from build123d import *

# Parameters (mm, degrees)
SKETCH1_R                 = 82
SKETCH1_R_2               = 75
BOSS_EXTRUDE1_DEPTH       = 9
SKETCH2_R                 = 5
CUT_EXTRUDE1_DEPTH        = 117.314229568
CIRPATTERN1_COUNT         = 4
M2X0_4_TAPPED_HOLE1_D     = 1.6
M2X0_4_TAPPED_HOLE1_DEPTH = 10
M2X0_4_TAPPED_HOLE1_TIP   = 0.480688495


with BuildPart() as part:
    # Sketch1 → Boss-Extrude1 (new body)
    with BuildSketch(Plane.XY):
        Circle(SKETCH1_R)
        Circle(SKETCH1_R_2, mode=Mode.SUBTRACT)
    extrude(amount=BOSS_EXTRUDE1_DEPTH)

    # Sketch2 → Cut-Extrude1 (cut, through all)
    with BuildSketch(Plane.XY.offset(9)):
        with Locations((0, 83)):
            Circle(SKETCH2_R)
    cut_extrude1 = extrude(amount=-CUT_EXTRUDE1_DEPTH, mode=Mode.SUBTRACT)

    # CirPattern1: Cut-Extrude1 ×4 about axis
    cirpattern1_axis = Axis((0, 0, 0), (0, 0, 1))
    for i in range(1, CIRPATTERN1_COUNT):
        add(cut_extrude1.rotate(cirpattern1_axis, i * 360 / CIRPATTERN1_COUNT), mode=Mode.SUBTRACT)

    # M2x0.4 Tapped Hole1
    with Locations(Plane(origin=(41, 71.01408311, 4.5), x_dir=(0.866025403784, -0.5, 0), z_dir=(0.5, 0.866025403784, 0))):
        with Locations((0, 0)):
            Hole(M2X0_4_TAPPED_HOLE1_D / 2, depth=M2X0_4_TAPPED_HOLE1_DEPTH)
            with Locations((0, 0, -(M2X0_4_TAPPED_HOLE1_DEPTH + M2X0_4_TAPPED_HOLE1_TIP / 2))):  # 118° drill point
                Cone(0, M2X0_4_TAPPED_HOLE1_D / 2, M2X0_4_TAPPED_HOLE1_TIP, mode=Mode.SUBTRACT)


solid = part.part
Work out the finished part from the listing and answer in its coordinate system (mm). Round coordinates to 2 decimals unless told otherwise and drop trailing zeros. Loops run counter-clockwise (first coordinate to the right, second up) from the corner with the lowest first, then second, coordinate; pieces in that order, holes last. Notation, with made-up numbers: M 83,36.25 L 104,36.25 A4 cw 104,42.25 Z; hole C 43.5,-8.5 d6. An arc over 180 degrees is marked long. One line per question, with ' | ' between items. Start each with the question number.
(1) Find the intervals of material crossed by line 1 (X direction, y = -14.5, z = 7.75); line 2 (X direction, y = 28, z = 6); line 3 (Y direction, x = -47, z = 8.5), in increasing order.
(2) Flat-ended cylindrical pins translate along their axes: pin 1 Ø5 at (x, z) = (29.5, 8) entering from +Y; pin 2 Ø1.5 at (x, z) = (-48, 4) entering from -Y; pin 3 Ø3 at (y, z) = (-35, 2.5) entering from -X. Find the tip coordinate at first contact, or state that the pin passes through.
(3) A cutting plane is placed at A-A on x = 0. Write down the section's boundary in (y, z).
(4) For a pull along Y with two mould halves and no side action, classify faces 1 (the face through (57.39, -58.57, 4.44)), 2 (the face through (58.57, 57.39, 4.44)), 3 (the face through (-78, 0, 5)) as released by +Y, released by -Y, zero draft, split by the parting line, or undercut.
(5) A cutting plane is placed at C-C on z = 7.5. Write down the section's boundary in (x, y).
Geometry check:
1) line 1: x = -80.71 to -73.58, 73.58 to 80.71 | line 2: x = -77.07 to -69.58, 69.58 to 77.07 | line 3: y = -67.19 to -58.45, 58.45 to 67.19
2) pin 1: stops at y = 77.43 | pin 2: stops at y = -67.02 | pin 3: stops at x = -74.84
3) outline: M -78,0 L -75,0 L -75,9 L -78,9 Z; M 75,0 L 78,0 L 78,9 L 75,9 Z
4) face 1: released by -Y | face 2: released by +Y | face 3: undercut
5) outline: M -81.86,-4.87 A82 ccw -4.87,-81.86 A5 cw 4.87,-81.86 A82 ccw 81.86,-4.87 A5 cw 81.86,4.87 A82 ccw 4.87,81.86 A5 cw -4.87,81.86 A82 ccw -81.86,4.87 A5 cw Z; hole C 0,0 d150
